The listing builds one solid part. Answer for the finished solid, in the listing's coordinates (mm). A direction names the side the tool comes from. Round coordinates to 2 decimals unless told otherwise and drop trailing zeros. Write each loop counter-clockwise with the first axis right and the second up, starting at its lowest first coordinate (ties: lowest second). Pieces come first, ordered by that corner, then holes.
Item 1: Each of these flat-tipped pins is pushed along its axis until it touches: pin 1 (3 mm diameter, centred on y = 38.5, z = 7.5, fed in from +X); pin 2 (5 mm diameter, centred on x = 11.5, y = 29, fed in from -Z); pin 3 (5 mm diameter, centred on x = 29.5, z = 3.5, fed in from +Y). Where does it stop, or does it pass through?
Item 2: A tool of negligible diameter and unlimited length cuts with its end or side. For faces 1 (the face through (0.86, 59.1, 5.07)), 2 (the face through (10, 33, 5)), from which of +Z, -Z, +X, -X, +Y, -Y can it reach the whole face along a straight path? Write none if from no direction.
Item 3: Find section A-A on x = 6. Give the vertices of the cut face in (y, z), then the cut area to 3 significant figures.
Item 4: Find section D-D on y = 16.5. Give the vertices of the cut face in (x, z), then the cut area to 3 significant figures.
Item 5: Find section B-B on z = 5. Give the vertices of the cut face in (x, y), then the cut area to 3 significant figures.
Item 6: Find the intervals of material crossed by probe 1 along Y at (x, z) = (40, 6.25); probe 2 along Y at (x, z) = (6, 3.5); probe 3 along Y at (x, z) = (20, 5.75), in increasing order.
Item 7: For a pull along Y with two mould halves and no side action, classify faces 3 (the face through (34, 10, 5)), 4 (the face through (0, 30, 5)), 5 (the face through (38.526, 7.352, 4.19)) as +Y half, -Y half, draft (parallel to the pull), parting line (faces both ways), or undercut.
```python
from build123d import *

# Parameters (mm, degrees)
F0_R     = 2
F1_DEPTH = 10
F2_R     = 3
F3_SIZE  = 1.5


with BuildPart() as f1:
    # F0 (on Top) → F1 (new body)
    with BuildSketch(Plane.XY):
        Polygon((0, 60), (0, 0), (60, 0), (60, 10), (10, 10), (10, 60), align=None)
        with Locations((40, 6)):
            Circle(F0_R, mode=Mode.SUBTRACT)
        with Locations((6, 40)):
            Circle(F0_R, mode=Mode.SUBTRACT)
    extrude(amount=F1_DEPTH)

    # F2
    f2_edges = [f1.edges().sort_by_distance(p)[0] for p in [
        (0, 0, 5),
        (60, 0, 5),
        (60, 10, 5),
        (10, 60, 5),
        (0, 60, 5),
    ]]
    fillet(f2_edges, radius=F2_R)

    # F3
    f3_edges = [f1.edges().sort_by_distance(p)[0] for p in [
        (4, 40, 10),
        (38, 6, 10),
    ]]
    chamfer(f3_edges, length=F3_SIZE)


solid = f1.part
```
Check values:
1. pin 1: stops at x = 10
1. pin 2: stops at z = 0
1. pin 3: stops at y = 10
2. face 1: +Z, -Z, -X, +Y
2. face 2: +Z, -Z, +X, +Y
3. outline: (0, 0) - (38, 0) - (38, 8.5) - (36.5, 10) - (0, 10) - close; (42, 0) - (60, 0) - (60, 10) - (43.5, 10) - (42, 8.5) - close
3. area: 558 mm2
4. outline: (0, 0) - (10, 0) - (10, 10) - (0, 10) - close
4. area: 100 mm2
5. outline: (0, 3) arc R3 ccw to (3, 0) - (57, 0) arc R3 ccw to (60, 3) - (60, 7) arc R3 ccw to (57, 10) - (10, 10) - (10, 57) arc R3 ccw to (7, 60) - (3, 60) arc R3 ccw to (0, 57) - close; hole circle Ø4 at (6, 40); hole circle Ø4 at (40, 6)
5. area: 1,070 mm2
6. probe 1: y = 0 to 4, 8 to 10
6. probe 2: y = 0 to 38, 42 to 60
6. probe 3: y = 0 to 10
7. face 3: +Y half
7. face 4: draft
7. face 5: undercut
